Design review of the part built by this model. Coordinates are the model's own, in mm. A direction names the side the tool comes from. Coordinates: 2 decimals unless noted, no trailing zeros. Loops run counter-clockwise (first coordinate to the right, second up) from the corner with the lowest first, then second, coordinate; pieces in that order, holes last. Notation, with made-up numbers: (-26.75, 6.5) - (20.25, 6.5) arc R25 ccw to (20.25, 27.5) - close; hole circle Ø2 at (20.25, 60). An arc over 180 degrees is marked (long way). Use one line per item in the form item = value. Start each with the question number.
(1) The part is to be moulded in two halves that separate along X. For faces 1 (the face through (9.5, 1, 0)), 2 (the face through (31, 9, 0)), 3 (the face through (0, 9, 10)), say which applies: pulls with the +X half, pulls with the -X half, needs draft (parallel to the pull), parting line crosses it, or undercut.
(2) Add section C-C (y = 16). State the section outline as (x, z) points, plus the area to 3 significant figures.
(3) Tool access review of faces 4 (the face through (-24, 0, 0)), 5 (the face through (0, 9, -10)), 6 (the face through (4, 9.6, -1.6)), 7 (the face through (-29, 13, 0)), 8 (the face through (12, 2, 0)): name each direction out of +Z, -Z, +X, -X, +Y, -Y from which nothing blocks a thin tool from reaching the whole face with its end or side.
(4) Add section D-D (x = -14.5). State the section outline as (y, z) points.
(5) Add section A-A (x = -1). State the section outline as (y, z) points, plus the area to 3 significant figures.
(6) Clearance check with flat-ended pins moving along their axes: pin 1 Ø3 at (x, z) = (-29.5, 1.5) entering from +Y; pin 2 Ø6 at (x, z) = (16, -7) entering from -Y; pin 3 Ø1.6 at (x, z) = (-10, -0.5) entering from -Y; pin 4 Ø4.5 at (x, z) = (-21, 0) entering from +Y. State where each tip first meets the part, or that it passes through.
(7) For L1, parallel to X at y = 3.8, z = 0; L2, parallel to X at y = 1.55, z = 0; L3, parallel to X at y = 10.5, z = 0, list the stretches that pass through material, from the lowest coordinate up.
(8) Add section B-B (z = 0). Count the separate pieces of the cut face and the enclosed holes in it, plus the area to 3 significant figures.
```python
from build123d import *

# Parameters (mm, degrees)
SKETCH1_W           = 62
SKETCH1_H           = 20
BOSS_EXTRUDE1_DEPTH = 13
BOSS_EXTRUDE2_DEPTH = 62
SKETCH3_W           = 2
SKETCH3_H           = 20
BOSS_EXTRUDE3_DEPTH = 4.8
SKETCH6_R           = 2.75
CUT_EXTRUDE1_DEPTH  = 14
CUT_EXTRUDE2_START  = 6
SKETCH7_R           = 5.25
CUT_EXTRUDE2_DEPTH  = 12.8
SKETCH8_W           = 5.5
SKETCH8_H           = 2
CUT_EXTRUDE3_DEPTH  = 21


with BuildPart() as part:
    # Sketch1 → Boss-Extrude1 (new body)
    with BuildSketch(Plane(origin=(0, 0, 0), x_dir=(1, 0, 0), z_dir=(0, 1, 0))):
        Rectangle(SKETCH1_W, SKETCH1_H)
    extrude(amount=BOSS_EXTRUDE1_DEPTH)

    # Sketch2 → Boss-Extrude2 (add)
    with BuildSketch(Plane.ZY.offset(31)):
        Polygon((3.2, 13), (8, 17.8), (10, 17.8), (10, 13), align=None)
        Polygon((-10, 13), (-3.2, 13), (-8, 17.8), (-10, 17.8), align=None)
    extrude(amount=-BOSS_EXTRUDE2_DEPTH)

    # Sketch3 → Boss-Extrude3 (add)
    with BuildSketch(Plane(origin=(0, 13, 0), x_dir=(1, 0, 0), z_dir=(0, 1, 0))):
        with Locations((30, 0)):
            Rectangle(SKETCH3_W, SKETCH3_H)
    extrude(amount=BOSS_EXTRUDE3_DEPTH)

    # Sketch6 → Cut-Extrude1 (cut, through all)
    with BuildSketch(Plane(origin=(0, 13, 0), x_dir=(1, 0, 0), z_dir=(0, 1, 0))):
        with Locations((-21, 0)):
            Circle(SKETCH6_R)
        with Locations((-1, 0)):
            Circle(SKETCH6_R)
    extrude(amount=-CUT_EXTRUDE1_DEPTH, mode=Mode.SUBTRACT)

    # Sketch7 → Cut-Extrude2 (cut, through all)
    with BuildSketch(Plane(origin=(0, 0, 0), x_dir=(1, 0, 0), z_dir=(0, 1, 0)).offset(CUT_EXTRUDE2_START)):
        with Locations((-21, 0)):
            Circle(SKETCH7_R)
        with Locations((-1, 0)):
            Circle(SKETCH7_R)
    extrude(amount=CUT_EXTRUDE2_DEPTH, mode=Mode.SUBTRACT)

    # Sketch8 → Cut-Extrude3 (cut, through all)
    with BuildSketch(Plane(origin=(0, 0, -10), x_dir=(-1, 0, 0), z_dir=(0, 0, -1))):
        with Locations((-12.25, 1)):
            Rectangle(SKETCH8_W, SKETCH8_H)
        with Locations((11, 1)):
            Rectangle(SKETCH8_W, SKETCH8_H)
    extrude(amount=-CUT_EXTRUDE3_DEPTH, mode=Mode.SUBTRACT)


solid = part.part
```
Computed values:
q1.face_1 = undercut
q1.face_2 = pulls with the +X half
q1.face_3 = needs draft
q2.outline = (-31, -10) - (31, -10) - (31, 10) - (-31, 10) - (-31, 6.2) - (29, 6.2) - (29, -6.2) - (-31, -6.2) - close
q2.area = 496 mm^2
q3.face_4 = +Z, -Z, +X, -X, -Y
q3.face_5 = -Z, +X, -X, +Y, -Y
q3.face_6 = +Y
q3.face_7 = -X, +Y
q3.face_8 = +Z, -Z, -Y
q4.outline = (0, -10) - (17.8, -10) - (17.8, -8) - (13, -3.2) - (13, 3.2) - (17.8, 8) - (17.8, 10) - (0, 10) - close
q5.outline = (0, -10) - (17.8, -10) - (17.8, -8) - (15.05, -5.25) - (6, -5.25) - (6, -2.75) - (0, -2.75) - close; (0, 2.75) - (6, 2.75) - (6, 5.25) - (15.05, 5.25) - (17.8, 8) - (17.8, 10) - (0, 10) - close
q5.area = 192 mm^2
q6.pin_1 = 13
q6.pin_2 = 0
q6.pin_3 = 2
q6.pin_4 = through
q7.L1 = -31 to -23.75, -18.25 to -3.75, 1.75 to 31
q7.L2 = -31 to -23.75, -18.25 to -13.75, -8.25 to -3.75, 1.75 to 9.5, 15 to 31
q7.L3 = -31 to -26.25, -15.75 to -6.25, 4.25 to 31
q8.separate_pieces = 3
q8.enclosed_holes = 0
q8.area = 581 mm^2
